Input: part model. Units: mm. Frame: model coordinates. A direction names the side the tool comes from. Round coordinates to 2 decimals unless told otherwise and drop trailing zeros. Loops run counter-clockwise (first coordinate to the right, second up) from the corner with the lowest first, then second, coordinate; pieces in that order, holes last.
1) First-contact query: pin 1 (1 mm diameter, centred on y = 16, z = 0.5, fed in from +X); pin 2 (4 mm diameter, centred on y = 19, z = 15.5, fed in from -X); pin 3 (3 mm diameter, centred on x = 3.5, z = -17.5, fed in from -Y); pin 4 (24.5 mm diameter, centred on x = 0, z = 0, fed in from -Y). Flat tips, straight axial feed; report the tip coordinate or a pass-through.
2) Draft query along X for faces 1 (the face through (13.48, 8.08, 42.81)), 2 (the face through (0.92, -25.03, -20.96)), 3 (the face through (-44, 13.144, 11)). Return one class per face: pulls with the +X half, pulls with the -X half, needs draft (parallel to the pull), parting line crosses it, or undercut.
3) Access query for faces 4 (the face through (11, -18.771, 11)), 5 (the face through (0.92, 25.21, -20.96)), 6 (the face through (-44, -13.144, -11)). Directions: +Z, -Z, +X, -X, +Y, -Y. A direction counts if a zero-diameter tool reaches every point of the face in a straight line with its end or side. Return the directions, or none.
4) Section B-B, the plane y = 25.5. Return loops of the section in (x, z).
5) Section A-A, the plane y = 15. Return loops of the section in (x, z), and give its area (3 significant figures).
6) Ray query, line 1 along Y through (x, z) = (36, 5); line 2 along X through (y, z) = (-21, -12.5); line 3 along Y through (x, z) = (8, 15). Return the intervals inside material, ascending.
from build123d import *

# Parameters (mm, degrees)
F2_SIZE = 0.762
F3_R    = 0.254


with BuildPart() as f1:
    # F0 (on Right) → F1 (revolve)
    with BuildSketch(Plane.YZ):
        Polygon((-18.7706, 15.1765), (0, 15.1765), (18.7706, 15.1765), (18.7706, 20.9804), (31.4706, 20.9804), (31.4706, 49.3522), (13.1445, 49.3522), (13.1445, 44.8818), (2.39395, 44.8818), (2.39395, 32.1818), (-2.39395, 32.1818), (-2.39395, 44.8818), (-13.1445, 44.8818), (-13.1445, 49.3522), (-31.4706, 49.3522), (-31.4706, 20.9804), (-18.7706, 20.9804), align=None)
    revolve(axis=Axis((0, -0.984378, 0), (0, 1, 0)))

    # F2
    f2_edges = [f1.edges().sort_by_distance(p)[0] for p in [
        (0, 2.39395, -44.8818),
        (0, -2.39395, -44.8818),
    ]]
    chamfer(f2_edges, length=F2_SIZE)

    # F3
    f3_edges = [f1.edges().sort_by_distance(p)[0] for p in [
        (0, 2.39395, -32.1818),
        (0, -2.39395, -32.1818),
    ]]
    fillet(f3_edges, radius=F3_R)


solid = f1.part
Final values:
1. pin 1: stops at x = 49.35
1. pin 2: stops at x = -47.47
1. pin 3: stops at y = -18.77
1. pin 4: passes through
2. face 1: parting line crosses it
2. face 2: undercut
2. face 3: needs draft
3. face 4: -Y
3. face 5: +Y
3. face 6: none
4. outline: circle Ø98.7 at (0, 0); hole circle Ø41.96 at (0, 0)
5. outline: circle Ø98.7 at (0, 0); hole circle Ø30.35 at (0, 0)
5. area: 6,930 mm2
6. line 1: y = -31.47 to -2.39, 2.39 to 31.47
6. line 2: x = -47.74 to -16.85, 16.85 to 47.74
6. line 3: y = -18.77 to 18.77
